from build123d import *

# Parameters (mm, degrees)
SKETCH1_R           = 4.25
BOSS_EXTRUDE1_DEPTH = 2
CUT_EXTRUDE1_DEPTH  = 5
CIRPATTERN1_COUNT   = 4
SKETCH3_R           = 1.5
CUT_EXTRUDE2_DEPTH  = 5
SKETCH5_R           = 1.85
CUT_EXTRUDE3_DEPTH  = 5


with BuildPart() as part:
    # Sketch1 → Boss-Extrude1 (new body)
    with BuildSketch(Plane(origin=(0, 0, 0), x_dir=(1, 0, 0), z_dir=(0, 1, 0))):
        with BuildLine():
            Line((-29, -34), (-25, -34))
            ThreePointArc((-25, -34), (-22.878679656, -33.121320344), (-22, -31))
            Line((-22, -31), (-22, -24.494897428))
            ThreePointArc((-22, -24.494897428), (-22.222539701, -23.361004009), (-22.857142857, -22.395334791))
            ThreePointArc((-22.857142857, -22.395334791), (-32, 0), (-22.857142857, 22.395334791))
            ThreePointArc((-22.857142857, 22.395334791), (-22.222539701, 23.361004009), (-22, 24.494897428))
            Line((-22, 24.494897428), (-22, 31))
            ThreePointArc((-22, 31), (-22.878679656, 33.121320344), (-25, 34))
            Line((-25, 34), (-29, 34))
            ThreePointArc((-29, 34), (-31.121320344, 34.878679656), (-32, 37))
            Line((-32, 37), (-32, 44))
            Line((-32, 44), (32, 44))
            Line((32, 44), (32, 37))
            ThreePointArc((32, 37), (31.121320344, 34.878679656), (29, 34))
            Line((29, 34), (25, 34))
            ThreePointArc((25, 34), (22.878679656, 33.121320344), (22, 31))
            Line((22, 31), (22, 24.494897428))
            ThreePointArc((22, 24.494897428), (22.222539701, 23.361004009), (22.857142857, 22.395334791))
            ThreePointArc((22.857142857, 22.395334791), (32, 0), (22.857142857, -22.395334791))
            ThreePointArc((22.857142857, -22.395334791), (22.222539701, -23.361004009), (22, -24.494897428))
            Line((22, -24.494897428), (22, -31))
            ThreePointArc((22, -31), (22.878679656, -33.121320344), (25, -34))
            Line((25, -34), (29, -34))
            ThreePointArc((29, -34), (31.121320344, -34.878679656), (32, -37))
            Line((32, -37), (32, -44))
            Line((32, -44), (-32, -44))
            Line((-32, -44), (-32, -37))
            ThreePointArc((-32, -37), (-31.121320344, -34.878679656), (-29, -34))
        make_face()
        with Locations(Location((0, 0, 0), (0, 0, 270))):
            Circle(SKETCH1_R, mode=Mode.SUBTRACT)
    extrude(amount=BOSS_EXTRUDE1_DEPTH)

    # Sketch2 → Cut-Extrude1 (cut)
    with BuildSketch(Plane(origin=(0, 2, 0), x_dir=(1, 0, 0), z_dir=(0, 1, 0))):
        with BuildLine():
            ThreePointArc((-11.674129624, 22.106892534), (-9.194159134, 22.25327912), (-7.454156207, 20.48012586))
            Line((-7.454156207, 20.48012586), (-6.070255366, 16.677889548))
            ThreePointArc((-6.070255366, 16.677889548), (-6.073907786, 14.615788781), (-7.40777769, 13.043190932))
            ThreePointArc((-7.40777769, 13.043190932), (-10.606601718, 10.606601718), (-13.043190932, 7.40777769))
            ThreePointArc((-13.043190932, 7.40777769), (-14.615788781, 6.073907786), (-16.677889548, 6.070255366))
            Line((-16.677889548, 6.070255366), (-20.48012586, 7.454156207))
            ThreePointArc((-20.48012586, 7.454156207), (-22.25327912, 9.194159134), (-22.106892534, 11.674129624))
            ThreePointArc((-22.106892534, 11.674129624), (-17.67766953, 17.67766953), (-11.674129624, 22.106892534))
        make_face()
    cut_extrude1 = extrude(amount=-CUT_EXTRUDE1_DEPTH, mode=Mode.SUBTRACT)

    # CirPattern1: Cut-Extrude1 ×4 about axis
    cirpattern1_axis = Axis((0, 0, 0), (0, 1, 0))
    for i in range(1, CIRPATTERN1_COUNT):
        add(cut_extrude1.rotate(cirpattern1_axis, i * 360 / CIRPATTERN1_COUNT), mode=Mode.SUBTRACT)

    # Sketch3 → Cut-Extrude2 (cut)
    with BuildSketch(Plane(origin=(0, 2, 0), x_dir=(1, 0, 0), z_dir=(0, 1, 0))):
        with Locations(Location((-8.5, 0, 0), (0, 0, 270))):
            Circle(SKETCH3_R)
        with Locations(Location((8.5, 0, 0), (0, 0, 270))):
            Circle(SKETCH3_R)
    extrude(amount=-CUT_EXTRUDE2_DEPTH, mode=Mode.SUBTRACT)

    # Sketch5 → Cut-Extrude3 (cut)
    with BuildSketch(Plane(origin=(0, 2, 0), x_dir=(1, 0, 0), z_dir=(0, 1, 0))):
        with Locations(Location((25, 38.82, 0), (0, 0, 270))):
            Circle(SKETCH5_R)
        with Locations(Location((-25, 38.82, 0), (0, 0, 270))):
            Circle(SKETCH5_R)
        with Locations(Location((-25, -38.82, 0), (0, 0, 270))):
            Circle(SKETCH5_R)
        with Locations(Location((25, -38.82, 0), (0, 0, 270))):
            Circle(SKETCH5_R)
    extrude(amount=-CUT_EXTRUDE3_DEPTH, mode=Mode.SUBTRACT)


solid = part.part
The model under review builds one solid part; all positions refer to its coordinate system, in mm. A direction names the side the tool comes from. Round coordinates to 2 decimals unless told otherwise and drop trailing zeros. Order: outer loops, then holes, each group sorted by start corner. A loop starts at its lowest first (then second) coordinate and runs counter-clockwise, first axis right, second up. Notation, with made-up numbers: (-23, 86.25) - (20, 86.25) arc R23 cw to (20, 104.25) - close; hole circle Ø4 at (83, 70.25). An arc over 180 degrees is marked (long way). Use one line per item in the form item = value.
Q1. Mouldability with a two-part tool opening along X and no side actions: class faces 4 (the cylindrical face through (-23.166, 1.014, -39.061)), 5 (the flat face through (27, 1, 34)), 6 (the flat face through (-32, 1, -40)) as pulls with the +X half, pulls with the -X half, needs draft (parallel to the pull), parting line crosses it, or undercut.
Response values:
face_4 = undercut
face_5 = needs draft
face_6 = pulls with the -X half
Q2. To check wall thickness, follow line 1 (X direction, y = 1.15, z = -38.82); line 2 (Z direction, x = -11, y = 1.6); line 3 (Z direction, x = -15, y = 0.3). State the ranges of each line that lie inside material, in increasing order.
Response values:
line_1 = -32 to -26.85, -23.15 to 23.15, 26.85 to 32
line_2 = -44 to -22.36, -10.2 to 10.2, 22.36 to 44
line_3 = -44 to -20, -5.96 to 5.96, 20 to 44
Q3. Add section D-D on y = 1.7. Give the number of separate pieces and of enclosed holes in the cut face, then the cut area to 3 significant figures.
Response values:
separate_pieces = 1
enclosed_holes = 11
area = 4,130 mm^2
Q4. Clearance check with flat-ended pins moving along their axes: P1, Ø1, axis at y = 1, z = 26.5, coming from the -X side; P2, Ø2, axis at x = -25, z = 38.82, coming from the -Y side; P3, Ø0.6, axis at y = 1, z = 29, coming from the +X side. State where each tip first meets the part, or that it passes through.
Response values:
P1 = -22
P2 = through
P3 = 22
Q5. Tool access review of faces 1 (the flat face through (27, 1, -34)), 2 (the flat face through (-6.75, 1.01, 18.55)), 3 (the flat face through (-22, 1, -28)): name each direction out of +Z, -Z, +X, -X, +Y, -Y from which nothing blocks a thin tool from reaching the whole face with its end or side.
Response values:
face_1 = +X, +Y, -Y
face_2 = +Y, -Y
face_3 = -X, +Y, -Y
Q6. Add section C-C on x = -8.5. Give the boundary of the cut face in (y, z).
Response values:
outline = (0, -44) - (2, -44) - (2, -21.87) - (0, -21.87) - close; (0, -12.36) - (2, -12.36) - (2, -1.5) - (0, -1.5) - close; (0, 1.5) - (2, 1.5) - (2, 12.36) - (0, 12.36) - close; (0, 21.87) - (2, 21.87) - (2, 44) - (0, 44) - close
Q7. Add section B-B on z = 38.82. Give the boundary of the cut face in (x, y).
Response values:
outline = (-32, 0) - (-26.85, 0) - (-26.85, 2) - (-32, 2) - close; (-23.15, 0) - (23.15, 0) - (23.15, 2) - (-23.15, 2) - close; (26.85, 0) - (32, 0) - (32, 2) - (26.85, 2) - close
Q8. Add section A-A on x = 0. Give the boundary of the cut face in (y, z).
Response values:
outline = (0, -44) - (2, -44) - (2, -4.25) - (0, -4.25) - close; (0, 4.25) - (2, 4.25) - (2, 44) - (0, 44) - close
